Source: CAD feature listing. Evaluate the final solid. Frame: model axes, mm. Round coordinates to 2 decimals unless told otherwise and drop trailing zeros. Write each loop counter-clockwise with the first axis right and the second up, starting at its lowest first coordinate (ties: lowest second). Pieces come first, ordered by that corner, then holes.
```python
from build123d import *

# Parameters (mm, degrees)
ESQUISSE1_W        = 100
ESQUISSE1_H        = 80
ESQUISSE1_R        = 1.5
ESQUISSE1_W_2      = 4
ESQUISSE1_H_2      = 22
ESQUISSE1_W_3      = 40
ESQUISSE1_H_3      = 3
BOSS_EXTRU_1_DEPTH = 3
ESQUISSE2_R        = 1
BOSS_EXTRU_2_DEPTH = 5


with BuildPart() as part:
    # Esquisse1 → Boss.-Extru.1 (new body)
    with BuildSketch(Plane.XY):
        Rectangle(ESQUISSE1_W, ESQUISSE1_H)
        with Locations((-46, 36)):
            Circle(ESQUISSE1_R, mode=Mode.SUBTRACT)
        with Locations((46, 36)):
            Circle(ESQUISSE1_R, mode=Mode.SUBTRACT)
        with Locations((46, -36)):
            Circle(ESQUISSE1_R, mode=Mode.SUBTRACT)
        with Locations((-46, -36)):
            Circle(ESQUISSE1_R, mode=Mode.SUBTRACT)
        with Locations((-40, 0)):
            Rectangle(ESQUISSE1_W_2, ESQUISSE1_H_2, mode=Mode.SUBTRACT)
        with Locations((40, 0)):
            Rectangle(ESQUISSE1_W_2, ESQUISSE1_H_2, mode=Mode.SUBTRACT)
        with Locations((0, 30)):
            Rectangle(ESQUISSE1_W_3, ESQUISSE1_H_3, mode=Mode.SUBTRACT)
    extrude(amount=BOSS_EXTRU_1_DEPTH)

    # Esquisse2 → Boss.-Extru.2 (add)
    with BuildSketch(Plane.XY.offset(3)):
        with Locations((-29, 24.5)):
            Circle(ESQUISSE2_R)
        with Locations((29, 24.5)):
            Circle(ESQUISSE2_R)
        with Locations((29, -24.5)):
            Circle(ESQUISSE2_R)
        with Locations((-29, -24.5)):
            Circle(ESQUISSE2_R)
    extrude(amount=BOSS_EXTRU_2_DEPTH)


solid = part.part
```
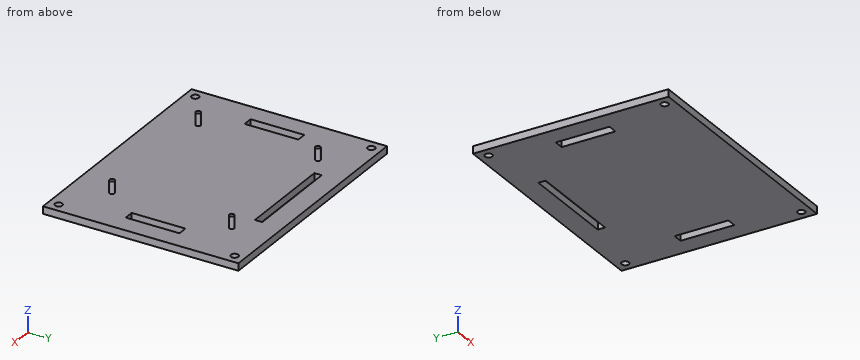
Q1. Section query B-B, the plane y = 36. Output: boundary loops of the cut face in (x, z).
Q2. Section query C-C, the plane x = 46. Output: boundary loops of the cut face in (y, z), and give its area (3 significant figures).
Q3. Line query: line 1 (Y direction, x = 46, z = 1.15); line 2 (X direction, y = 7.5, z = 1.75); line 3 (Y direction, x = 13, z = 0.5). Output: solid intervals per line, ascending.
Q4. Section query A-A, the plane x = -40.5. Output: boundary loops of the cut face in (y, z).
Q5. Section query D-D, the plane z = 6.5. Output: boundary loops of the cut face in (x, y).
Q6. Pin query (flat end, axial travel): P1, Ø6, axis at x = -29, y = 2.5, coming from the +Z side. Return the tip coordinate at first contact, or that it passes through.
Filled in:
1. outline: (-50, 0) - (-47.5, 0) - (-47.5, 3) - (-50, 3) - close; (-44.5, 0) - (44.5, 0) - (44.5, 3) - (-44.5, 3) - close; (47.5, 0) - (50, 0) - (50, 3) - (47.5, 3) - close
2. outline: (-40, 0) - (-37.5, 0) - (-37.5, 3) - (-40, 3) - close; (-34.5, 0) - (34.5, 0) - (34.5, 3) - (-34.5, 3) - close; (37.5, 0) - (40, 0) - (40, 3) - (37.5, 3) - close
2. area: 222 mm2
3. line 1: y = -40 to -37.5, -34.5 to 34.5, 37.5 to 40
3. line 2: x = -50 to -42, -38 to 38, 42 to 50
3. line 3: y = -40 to 28.5, 31.5 to 40
4. outline: (-40, 0) - (-11, 0) - (-11, 3) - (-40, 3) - close; (11, 0) - (40, 0) - (40, 3) - (11, 3) - close
5. outline: circle Ø2 at (-29, -24.5); circle Ø2 at (-29, 24.5); circle Ø2 at (29, -24.5); circle Ø2 at (29, 24.5)
6. P1: stops at z = 3
